from build123d import *

# Parameters (mm, degrees)
F0_W     = 50
F0_H     = 30
F1_DEPTH = 40
F3_DEPTH = 50.001
F5_DEPTH = 40.001


with BuildPart() as f1:
    # F0 (on Front) → F1 (new body)
    with BuildSketch(Plane.XZ):
        Rectangle(F0_W, F0_H)
    extrude(amount=F1_DEPTH)

    # F2 (on face) → F3 (cut, through all)
    with BuildSketch(Plane(origin=(-25, 0, 0), x_dir=(0, -1, 0), z_dir=(-1, 0, 0))):
        Polygon((16, 5), (16, 10), (12.5, 10), (12.5, 15), (0, 15), (0, 5), align=None)
        Polygon((40, 15), (27.5, 15), (27.5, 10), (23.938067, 10), (24, 5), (40, 5), align=None)
    extrude(amount=-F3_DEPTH, mode=Mode.SUBTRACT)

    # F4 (on face) → F5 (cut, through all)
    with BuildSketch(Plane.XZ.offset(40)):
        Polygon((-7.5, -10), (-7.5, -15), (7.5, -15), (7.5, -10), (11.972041, -10), (11.972041, -5), (-13.027959, -5), (-13.027959, -10), align=None)
    extrude(amount=-F5_DEPTH, mode=Mode.SUBTRACT)


solid = f1.part
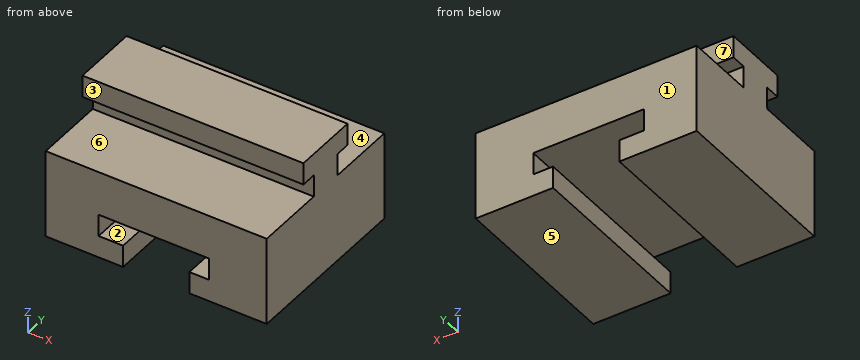
For this review, take the finished solid that the model builds, in its own axes (mm). Face numbers are marked on the shaded views. A direction names the side the tool comes from. Give positions to 0.01 mm unless a question says otherwise; leave off trailing zeros. Order: outer loops, then holes, each group sorted by start corner. A loop starts at its lowest first (then second) coordinate and runs counter-clockwise, first axis right, second up. Notation, with made-up numbers: (-12.5, -31.75) -> (14.5, -31.75) arc R18 cw to (14.5, -1.75) -> close; hole circle Ø6 at (76, 41). An arc over 180 degrees is marked (long way). Write item = value, one per line.
1) We need section A-A, the plane z = -8.5. Give the boundary of the cut face in (x, y).
Findings:
outline = (-25, -40) -> (-13.03, -40) -> (-13.03, 0) -> (-25, 0) -> close; (11.97, -40) -> (25, -40) -> (25, 0) -> (11.97, 0) -> close
2) We need section C-C, the plane x = 19. Give the boundary of the cut face in (y, z).
Findings:
outline = (-40, -15) -> (0, -15) -> (0, 5) -> (-16, 5) -> (-16, 10) -> (-12.5, 10) -> (-12.5, 15) -> (-27.5, 15) -> (-27.5, 10) -> (-23.94, 10) -> (-24, 5) -> (-40, 5) -> close
3) To check wall thickness, follow L1, parallel to Z at x = -20, y = -25.5; L2, parallel to Z at x = -2, y = -13; L3, parallel to X at y = -35, z = -12.75. State the ranges of each line that lie inside material, in increasing order. Write a range as from..to.
Findings:
L1 = -15..5, 10..15
L2 = -5..5, 10..15
L3 = -25..-7.5, 7.5..25
4) Insertion check: pin 1 (1.5 mm diameter, centred on x = -3.5, z = 8, fed in from +Y); pin 2 (5.5 mm diameter, centred on x = -6, z = 13.5, fed in from -Y); pin 3 (4 mm diameter, centred on x = -8.5, z = 13, fed in from +Y). Each pin has a flat end and moves straight along its axis. Give the tip position at first contact, or say it passes through.
Findings:
pin_1 = -16
pin_2 = -27.5
pin_3 = -12.5
5) For the marked faces 1, 2, 3 and 4, list the 3-axis set-ups (+Z, -Z, +X, -X, +Y, -Y) from which the entire face can be reached by the end or side of a thin tool; tool diameter is ignored.
Findings:
face_1 = +Z, -Z, +X, -X, +Y
face_2 = +Y, -Y
face_3 = +Z, +X, -X, -Y
face_4 = +X, -X, +Y
6) We need section B-B, the plane y = -13.5. Give the boundary of the cut face in (x, z), and give its area (3 significant figures).
Findings:
outline = (-25, -15) -> (-7.5, -15) -> (-7.5, -10) -> (-13.03, -10) -> (-13.03, -5) -> (11.97, -5) -> (11.97, -10) -> (7.5, -10) -> (7.5, -15) -> (25, -15) -> (25, 5) -> (-25, 5) -> close; (-25, 10) -> (25, 10) -> (25, 15) -> (-25, 15) -> close
area = 1,050 mm^2
7) Draft analysis for pull direction Z (two halves, no side actions). For the marked faces 5, 6 and 7, state which applies: pulls with the +Z half, pulls with the -Z half, needs draft (parallel to the pull), parting line crosses it, or undercut.
Findings:
face_5 = pulls with the -Z half
face_6 = undercut
face_7 = needs draft
8) We need section D-D, the plane y = -6. Give the boundary of the cut face in (x, z).
Findings:
outline = (-25, -15) -> (-7.5, -15) -> (-7.5, -10) -> (-13.03, -10) -> (-13.03, -5) -> (11.97, -5) -> (11.97, -10) -> (7.5, -10) -> (7.5, -15) -> (25, -15) -> (25, 5) -> (-25, 5) -> close
